Can you work these out from the model? Positions are in its coordinate system, mm. A direction names the side the tool comes from. Give positions to 0.01 mm unless a question says otherwise; leave off trailing zeros. Order: outer loops, then holes, each group sorted by start corner. A loop starts at its lowest first (then second) coordinate and runs counter-clockwise, first axis right, second up. Notation, with made-up numbers: (53, 19) - (106, 19) arc R25 cw to (106, 57) - close; hole circle Ø6 at (9.5, 44.25). An arc over 180 degrees is marked (long way). Use one line per item in the form item = value. Start each with the question number.
1) We'd pull the mould along X, two halves only. Please class faces 1 (the flat face through (-5.5, 25, 0)), 2 (the flat face through (-40.5, 17, -1)), 3 (the flat face through (-14, 26, -13.5)), 4 (the flat face through (-52, 6, 2)): released by +X, released by -X, zero draft, split by the parting line, or undercut.
2) Please list where these lines run through material, in increasing order: probe 1 along Y at (x, z) = (-11, -3); probe 2 along X at (y, z) = (16, -4.5); probe 3 along Z at (x, y) = (-41.75, 33).
3) Which directions (+Z, -Z, +X, -X, +Y, -Y) give clear straight access to the entire face, cutting with the end or side of a thin tool? Please do faces 5 (the flat face through (-31.5, 19, -7)), 6 (the cylindrical face through (-19.979, 16.892, -1.484)), 7 (the cylindrical face through (-42.472, 23.462, -3.414)).
4) Suppose I cut it at C-C, the plane z = 11.25. Write out the boundary of the cut face in (x, y), and give its area (3 significant figures).
5) For pin 1 (6 mm diameter, centred on y = 19, z = -2.83, fed in from -X); pin 2 (10.5 mm diameter, centred on y = 27, z = 1, fed in from +X); pin 3 (4 mm diameter, centred on x = -24, z = 5.5, fed in from +Y), each with a flat end and sliding along its axis, tell me the tip position at first contact or that it passes through.
6) Suppose I cut it at A-A, the plane z = -9.75. State how many separate pieces and enclosed holes the cut face has, and give its area (3 significant figures).
```python
from build123d import *

# Parameters (mm, degrees)
CROQUIS1_R              = 2.5
SALIENTE_EXTRUIR1_DEPTH = 10
CROQUIS6_R              = 5
CORTAR_EXTRUIR1_DEPTH   = 4
REDONDEO3_R             = 0.5
SALIENTE_EXTRUIR2_DEPTH = 30
CROQUIS8_W              = 16
CROQUIS8_H              = 22
SALIENTE_EXTRUIR3_DEPTH = 28
CROQUIS9_R              = 4.5
CORTAR_EXTRUIR2_DEPTH   = 4
CORTAR_EXTRUIR3_REACH   = 70.544
CROQUIS10_R             = 2.5
CORTAR_EXTRUIR4_START   = -4
CROQUIS11_R             = 4.5
CORTAR_EXTRUIR4_DEPTH   = 4
REDONDEO4_R             = 5
CROQUIS13_W             = 4
CROQUIS13_H             = 10
CORTAR_EXTRUIR6_DEPTH   = 17


with BuildPart() as part:
    # Croquis1 → Saliente-Extruir1 (new body)
    with BuildSketch(Plane(origin=(0, 0, 0), x_dir=(1, 0, 0), z_dir=(0, 1, 0))):
        with BuildLine():
            Line((0, -13.5), (-50, -13.5))
            ThreePointArc((-50, -13.5), (-63.5, 0), (-50, 13.5))
            Line((-50, 13.5), (0, 13.5))
            ThreePointArc((0, 13.5), (13.5, 0), (0, -13.5))
        make_face()
        with Locations(Location((-50, 0, 0), (0, 0, 270))):
            Circle(CROQUIS1_R, mode=Mode.SUBTRACT)
        with Locations(Location((0, 0, 0), (0, 0, 90))):
            Circle(CROQUIS1_R, mode=Mode.SUBTRACT)
    extrude(amount=SALIENTE_EXTRUIR1_DEPTH)

    # Croquis6 → Cortar-Extruir1 (cut, symmetric)
    with BuildSketch(Plane(origin=(0, 10, 0), x_dir=(1, 0, 0), z_dir=(0, 1, 0))):
        with Locations(Location((-50, 0, 0), (0, 0, 270))):
            Circle(CROQUIS6_R)
        with Locations(Location((0, 0, 0), (0, 0, 270))):
            Circle(CROQUIS6_R)
    extrude(amount=CORTAR_EXTRUIR1_DEPTH, both=True, mode=Mode.SUBTRACT)

    # Redondeo3
    redondeo3_edges = [part.edges().sort_by_distance(p)[0] for p in [
        (-50, 10, -5),
        (0, 10, -5),
    ]]
    fillet(redondeo3_edges, radius=REDONDEO3_R)

    # Croquis7 → Saliente-Extruir2 (add)
    with BuildSketch(Plane(origin=(0, 10, 0), x_dir=(1, 0, 0), z_dir=(0, 1, 0))):
        Polygon((-44.5, -8.5), (-5.5, -6.9), (-5.5, -13.5), (-44.5, -13.5), align=None)
    extrude(amount=SALIENTE_EXTRUIR2_DEPTH)

    # Croquis8 → Saliente-Extruir3 (add)
    with BuildSketch(Plane(origin=(0, 40, 0), x_dir=(1, 0, 0), z_dir=(0, 1, 0))):
        with Locations((-13.5, 2.5)):
            Rectangle(CROQUIS8_W, CROQUIS8_H)
        with Locations((-36.5, 2.5)):
            Rectangle(CROQUIS8_W, CROQUIS8_H)
    extrude(amount=-SALIENTE_EXTRUIR3_DEPTH)

    # Croquis9 → Cortar-Extruir2 (cut)
    with BuildSketch(Plane(origin=(-5.5, 0, 0), x_dir=(0, 0, -1), z_dir=(1, 0, 0))):
        with Locations((2.828205128, 33)):
            Circle(CROQUIS9_R)
        with Locations(Location((2.828205128, 19, 0), (0, 0, 180))):
            Circle(CROQUIS9_R)
    extrude(amount=-CORTAR_EXTRUIR2_DEPTH, mode=Mode.SUBTRACT)

    # Cortar-Extruir3: up to this face of the body (flat: up to its plane)
    cortar_extruir3_end = Plane(part.part.faces().sort_by_distance((-44.5, 25.804177546, 0.143603133))[0])
    # Croquis10 → Cortar-Extruir3 (cut, up to the picked face)
    with BuildSketch(Plane(origin=(-9.5, 0, 0), x_dir=(0, 0, -1), z_dir=(1, 0, 0)), mode=Mode.PRIVATE) as cortar_extruir3_sk1:
        with Locations((2.828205128, 33)):
            Circle(CROQUIS10_R)
    cortar_extruir3_tool1 = split(extrude(cortar_extruir3_sk1.sketch, amount=-CORTAR_EXTRUIR3_REACH, mode=Mode.PRIVATE), bisect_by=cortar_extruir3_end, keep=Keep.BOTH, mode=Mode.PRIVATE)
    # Croquis10 → Cortar-Extruir3 (cut, up to the picked face)
    with BuildSketch(Plane(origin=(-9.5, 0, 0), x_dir=(0, 0, -1), z_dir=(1, 0, 0)), mode=Mode.PRIVATE) as cortar_extruir3_sk2:
        with Locations(Location((2.828205128, 19, 0), (0, 0, 180))):
            Circle(CROQUIS10_R)
    cortar_extruir3_tool2 = split(extrude(cortar_extruir3_sk2.sketch, amount=-CORTAR_EXTRUIR3_REACH, mode=Mode.PRIVATE), bisect_by=cortar_extruir3_end, keep=Keep.BOTH, mode=Mode.PRIVATE)
    add(cortar_extruir3_tool1.solids().sort_by(Axis((-9.5, 33, -2.828205), (-1, 0, 0)))[0], mode=Mode.SUBTRACT)
    add(cortar_extruir3_tool2.solids().sort_by(Axis((-9.5, 19, -2.828205), (-1, 0, 0)))[0], mode=Mode.SUBTRACT)

    # Croquis11 → Cortar-Extruir4 (cut)
    with BuildSketch(Plane.ZY.offset(44.5).offset(CORTAR_EXTRUIR4_START)):
        with Locations(Location((-2.828205128, 33, 0), (0, 0, 180))):
            Circle(CROQUIS11_R)
        with Locations((-2.828205128, 19)):
            Circle(CROQUIS11_R)
    extrude(amount=CORTAR_EXTRUIR4_DEPTH, mode=Mode.SUBTRACT)

    # Redondeo4
    # the kernel refuses this fillet: 5 mm, written as the material it takes off along each edge
    with BuildSketch(Plane(origin=(-28.5, 40, 20.343589744), x_dir=(-1, 0, 0), z_dir=(0, 0, -1))) as redondeo4_piece_1_section:
        with BuildLine():
            CenterArc((REDONDEO4_R, -REDONDEO4_R), REDONDEO4_R, 90, 90)
            Line((0, -REDONDEO4_R), (0, 0))
            Line((0, 0), (REDONDEO4_R, 0))
        make_face()
    redondeo4_piece_1 = extrude(amount=46.343589744, mode=Mode.PRIVATE)
    redondeo4_piece_1 = split(redondeo4_piece_1, bisect_by=Plane(origin=(-29.180561705, 38.884335507, 7.871510224), z_dir=(-0.04099115935241428, 0, -0.9991595092150929)), keep=Keep.TOP, mode=Mode.PRIVATE)
    add(redondeo4_piece_1, mode=Mode.SUBTRACT)
    with BuildSketch(Plane(origin=(-21.5, 40, -26), x_dir=(1, 0, 0), z_dir=(0, 0, 1))) as redondeo4_piece_2_section:
        with BuildLine():
            CenterArc((REDONDEO4_R, -REDONDEO4_R), REDONDEO4_R, 90, 90)
            Line((0, -REDONDEO4_R), (0, 0))
            Line((0, 0), (REDONDEO4_R, 0))
        make_face()
    redondeo4_piece_2 = extrude(amount=46.056410256, mode=Mode.PRIVATE)
    redondeo4_piece_2 = split(redondeo4_piece_2, bisect_by=Plane(origin=(-19.954554265, 38.882337261, 7.493007354), z_dir=(-0.04099115935241428, 0, -0.9991595092150929)), keep=Keep.TOP, mode=Mode.PRIVATE)
    add(redondeo4_piece_2, mode=Mode.SUBTRACT)

    # Croquis13 → Cortar-Extruir6 (cut)
    with BuildSketch(Plane(origin=(0, 0, -13.5), x_dir=(-1, 0, 0), z_dir=(0, 0, -1))):
        with Locations((16.5, 33)):
            Rectangle(CROQUIS13_W, CROQUIS13_H)
        with Locations((16.5, 19)):
            Rectangle(CROQUIS13_W, CROQUIS13_H)
        with Locations((33.5, 19)):
            Rectangle(CROQUIS13_W, CROQUIS13_H)
        with Locations((33.5, 33)):
            Rectangle(CROQUIS13_W, CROQUIS13_H)
    extrude(amount=-CORTAR_EXTRUIR6_DEPTH, mode=Mode.SUBTRACT)


solid = part.part
```
Result sheet:
q1.face_1 = released by +X
q1.face_2 = released by -X
q1.face_3 = zero draft
q1.face_4 = undercut
q2.probe_1 = 0 to 10, 12 to 16.51, 21.49 to 30.51, 35.49 to 40
q2.probe_2 = -40.5 to -35.5, -31.5 to -28.5, -21.5 to -18.5, -14.5 to -9.5
q2.probe_3 = -13.5 to -7.33, 1.67 to 13.5
q3.face_5 = -Z
q3.face_6 = +X, -X
q3.face_7 = -X
q4.outline = (-57.46, 0) - (7.46, 0) - (7.46, 10) - (-5.5, 10) - (-5.5, 40) - (-44.5, 40) - (-44.5, 10) - (-57.46, 10) - close
q4.area = 1,820 mm²
q5.pin_1 = -40.5
q5.pin_2 = -5.5
q5.pin_3 = 10
q6.separate_pieces = 3
q6.enclosed_holes = 4
q6.area = 1,410 mm²
